The model under review builds one solid part; all positions refer to its coordinate system, in mm. Face numbers are marked on the shaded views. Coordinates: 2 decimals unless noted, no trailing zeros. Order: outer loops, then holes, each group sorted by start corner. A loop starts at its lowest first (then second) coordinate and runs counter-clockwise, first axis right, second up. Notation, with made-up numbers: (69.25, -24.75) -> (121.25, -24.75) arc R21 cw to (121.25, 9.25) -> close; hole circle Ø1 at (26.5, 16). An arc over 180 degrees is marked (long way). Use one line per item in the form item = value. Start each with the question number.
(1) Mouldability with a two-part tool opening along Y and no side actions: class the marked faces 1, 2, 3 and 4 as +Y half, -Y half, draft (parallel to the pull), parting line (faces both ways), or undercut.
(2) Take a section at A-A (x = 0). State the section outline as (y, z) points, then the cut area to 3 significant figures.
(3) Take a section at C-C (y = -0.5). State the section outline as (x, z) points.
(4) Insertion check: pin 1 Ø4.5 at (x, z) = (0, 8) entering from -Y; pin 2 Ø5 at (x, z) = (0, 0) entering from -Y; pin 3 Ø3 at (y, z) = (-2, 2) entering from -X. Each pin has a flat end and moves straight along its axis. Give the tip position at first contact, or say it passes through.
(5) Take a section at D-D (z = -8.5). State the section outline as (x, y) points, then the cut area to 3 significant figures.
(6) Wall thickness on line 1 along Z through (x, y) = (0, -3.45); line 2 along Y through (x, z) = (0, -11.5); line 3 along Z through (x, y) = (0, -6.3): over which ranges is each line inside the solid? List them lowest first.
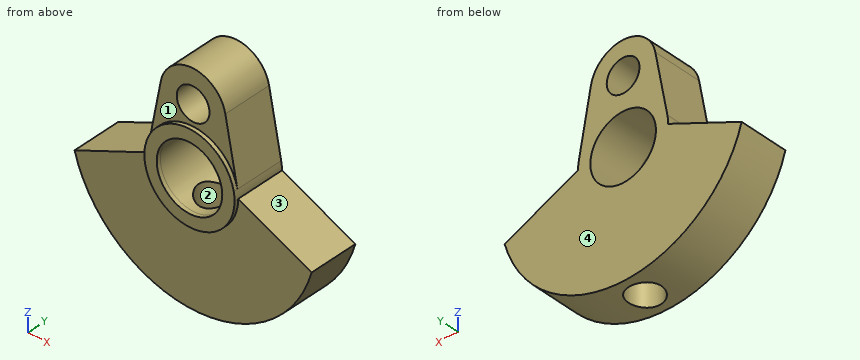
```python
from build123d import *

# Parameters (mm, degrees)
F0_R     = 2
F1_DEPTH = 6
F2_R     = 4
F3_DEPTH = 25
F4_R     = 4
F5_DEPTH = 0.5
F7_R     = 2
F8_DEPTH = 12.535898485


with BuildPart() as f1:
    # F0 (on Front) → F1 (new body)
    with BuildSketch(Plane.XZ):
        with BuildLine():
            Line((-5.5, 0), (-14.4568322948, -4))
            ThreePointArc((-14.4568322948, -4), (0, -15), (14.4568322948, -4))
            Line((14.4568322948, -4), (5.5, 0))
            ThreePointArc((5.5, 0), (5.4755595256, 0.5179265218), (5.4024553156, 1.03125))
            Line((5.4024553156, 1.03125), (3.9290584114, 8.75))
            ThreePointArc((3.9290584114, 8.75), (0, 12), (-3.9290584114, 8.75))
            Line((-3.9290584114, 8.75), (-5.4024553156, 1.03125))
            ThreePointArc((-5.4024553156, 1.03125), (-5.4755595256, 0.5179265218), (-5.5, 0))
        make_face()
        with Locations((0, 8)):
            Circle(F0_R, mode=Mode.SUBTRACT)
    extrude(amount=F1_DEPTH)

    # F2 (on face) → F3 (cut)
    with BuildSketch(Plane.XZ.offset(6)):
        Circle(F2_R)
    extrude(amount=-F3_DEPTH, mode=Mode.SUBTRACT)

    # F4 (on face) → F5 (join)
    with BuildSketch(Plane.XZ.offset(6)):
        with BuildLine():
            ThreePointArc((-5.5, 0), (0, -5.5), (5.5, 0))
            ThreePointArc((5.5, 0), (5.4755595256, 0.5179265218), (5.4024553156, 1.03125))
            ThreePointArc((5.4024553156, 1.03125), (0, 5.5), (-5.4024553156, 1.03125))
            ThreePointArc((-5.4024553156, 1.03125), (-5.4755595256, 0.5179265218), (-5.5, 0))
        make_face()
        Circle(F4_R, mode=Mode.SUBTRACT)
    extrude(amount=F5_DEPTH)

    # F7 (on offset) → F8 (cut, up to face)
    with BuildSketch(Plane.XY.offset(-15)):
        with Locations((0, -3)):
            Circle(F7_R)
    extrude(amount=F8_DEPTH, mode=Mode.SUBTRACT)


solid = f1.part
```
Findings:
q1.face_1 = -Y half
q1.face_2 = undercut
q1.face_3 = draft
q1.face_4 = +Y half
q2.outline = (-6.5, -5.5) -> (-6, -5.5) -> (-6, -15) -> (-5, -15) -> (-5, -4) -> (-6.5, -4) -> close; (-6.5, 4) -> (0, 4) -> (0, 6) -> (-6, 6) -> (-6, 5.5) -> (-6.5, 5.5) -> close; (-6, 10) -> (0, 10) -> (0, 12) -> (-6, 12) -> close; (-1, -15) -> (0, -15) -> (0, -4) -> (-1, -4) -> close
q2.area = 47.5 mm²
q3.outline = (-14.46, -4) arc R15 ccw to (14.46, -4) -> (5.5, 0) arc R5.5 ccw to (5.4, 1.03) -> (3.93, 8.75) arc R4 ccw to (-3.93, 8.75) -> (-5.4, 1.03) arc R5.5 ccw to (-5.5, 0) -> close; hole circle Ø8 at (0, 0); hole circle Ø4 at (0, 8)
q4.pin_1 = -6
q4.pin_2 = through
q4.pin_3 = -5.48
q5.outline = (-12.36, -6) -> (12.36, -6) -> (12.36, 0) -> (-12.36, 0) -> close; hole circle Ø4 at (0, -3)
q5.area = 136 mm²
q6.line_1 = 4 to 6, 10 to 12
q6.line_2 = -6 to -5, -1 to 0
q6.line_3 = -5.5 to -4, 4 to 5.5
